```python
from build123d import *

# Parameters (mm, degrees)
SKETCH2_R           = 15
SKETCH2_R_2         = 12.5
BOSS_EXTRUDE1_DEPTH = 35
SKETCH3_R           = 15
BOSS_EXTRUDE2_DEPTH = 5
SKETCH4_W           = 22.056214186
SKETCH4_H           = 2.649940184
BOSS_EXTRUDE3_DEPTH = 10
SKETCH5_W           = 4.385639536
SKETCH5_H           = 22.056214186
BOSS_EXTRUDE4_DEPTH = 40
FILLET1_R           = 2.5


with BuildPart() as part:
    # Sketch2 → Boss-Extrude1 (new body)
    with BuildSketch(Plane(origin=(0, 0, 0), x_dir=(1, 0, 0), z_dir=(0, 1, 0))):
        with Locations(Location((0, 0, 0), (0, 0, 270))):
            Circle(SKETCH2_R)
        with Locations(Location((0, 0, 0), (0, 0, 270))):
            Circle(SKETCH2_R_2, mode=Mode.SUBTRACT)
    extrude(amount=BOSS_EXTRUDE1_DEPTH)

    # Sketch3 → Boss-Extrude2 (add)
    with BuildSketch(Plane(origin=(0, 35, 0), x_dir=(1, 0, 0), z_dir=(0, 1, 0))):
        with Locations(Location((0, 0, 0), (0, 0, 270))):
            Circle(SKETCH3_R)
    extrude(amount=BOSS_EXTRUDE2_DEPTH)

    # Sketch4 → Boss-Extrude3 (add)
    with BuildSketch(Plane(origin=(10, 0, 0), x_dir=(0, 0, -1), z_dir=(1, 0, 0))):
        with Locations((0, 37.460010141)):
            Rectangle(SKETCH4_W, SKETCH4_H)
    extrude(amount=BOSS_EXTRUDE3_DEPTH)

    # Sketch5 → Boss-Extrude4 (add)
    with BuildSketch(Plane.XZ.offset(-36.135040049)):
        with Locations((17.807180232, 0)):
            Rectangle(SKETCH5_W, SKETCH5_H)
    extrude(amount=BOSS_EXTRUDE4_DEPTH)

    # Fillet1
    fillet1_edges = [part.edges().sort_by_distance(p)[0] for p in [
        (20, 17.460010141, -11.028107093),
        (20, 38.784980233, 0),
        (20, 17.460010141, 11.028107093),
        (20, -3.864959951, 0),
    ]]
    fillet(fillet1_edges, radius=FILLET1_R)


solid = part.part
```
Build history of the part. All positions in model axes, mm. A direction names the side the tool comes from. Round coordinates to 2 decimals unless told otherwise and drop trailing zeros. Write each loop counter-clockwise with the first axis right and the second up, starting at its lowest first coordinate (ties: lowest second). Pieces come first, ordered by that corner, then holes. Notation, with made-up numbers: (-26.75, 20) - (-17.75, 20) arc R27 cw to (-17.75, 43) - close; hole circle Ø11 at (-2, 87). An arc over 180 degrees is marked (long way). Write each question's results on one line, items separated by ' | '. Start each with the question number.
Item 1: Saw through at D-D (x = 13.5). Write the cut outline in (y, z).
Item 2: Saw through at B-B (x = 0). Write the cut outline in (y, z), and give its area (3 significant figures).
Item 3: Saw through at A-A (y = 5). Write the cut outline in (x, z), and give its area (3 significant figures).
Item 4: Drop flat-ended pins along their axis: P1, Ø1.6, axis at x = 12.5, z = -3.5, coming from the -Y side; P2, Ø1.5, axis at y = 9.5, z = 10, coming from the +X side; P3, Ø1, axis at x = 15.5, z = -1, coming from the +Y side (3 decimals); P4, Ø12, axis at y = 12.5, z = -5, coming from the -X side. Give the stop position or say it passes through.
Item 5: Saw through at C-C (z = 0). Write the cut outline in (x, y), and give its area (3 significant figures).
Item 6: Which spindle directions (+Z, -Z, +X, -X, +Y, -Y) get a long thin tool onto all of the face, cutting with end or side? Do faces 1 (the face through (15.614, 16, 0)), 2 (the face through (17, 21, 11.028)), 3 (the face through (3.755, 17.255, 11.923)). Say none if no direction does.
Item 7: Wall check: L1, parallel to X at y = 21, z = 0; L2, parallel to X at y = 17, z = -6.75; L3, parallel to Z at x = -0.5, y = 13.5. Give the ranges that are in metal, low to high. Write a range as [from, to].
Results are:
1) outline: (0, -6.54) - (36.14, -6.54) - (36.14, -11.03) - (38.78, -11.03) - (38.78, -6.54) - (40, -6.54) - (40, 6.54) - (38.78, 6.54) - (38.78, 11.03) - (36.14, 11.03) - (36.14, 6.54) - (0, 6.54) - close
2) outline: (0, -15) - (40, -15) - (40, 15) - (0, 15) - (0, 12.5) - (35, 12.5) - (35, -12.5) - (0, -12.5) - close | area: 325 mm²
3) outline: circle Ø30 at (0, 0); (15.61, -11.03) - (17.5, -11.03) arc R2.5 ccw to (20, -8.53) - (20, 8.53) arc R2.5 ccw to (17.5, 11.03) - (15.61, 11.03) - close; hole circle Ø25 at (0, 0) | area: 310 mm²
4) P1: stops at y = 0 | P2: stops at x = 19.89 | P3: stops at y = 38.785 | P4: stops at x = -15
5) outline: (-15, 0) - (-12.5, 0) - (-12.5, 35) - (12.5, 35) - (12.5, 0) - (15, 0) - (15, 36.14) - (15.61, 36.14) - (15.61, -3.86) - (17.5, -3.86) arc R2.5 ccw to (20, -1.36) - (20, 36.28) arc R2.5 ccw to (17.5, 38.78) - (15, 38.78) - (15, 40) - (-15, 40) - close | area: 511 mm²
6) face 1: +Z, -Z, -Y | face 2: +Z, +X, +Y, -Y | face 3: -Y
7) L1: x = [-15, -12.5], [12.5, 15], [15.61, 20] | L2: x = [-13.4, -10.52], [10.52, 13.4], [15.61, 20] | L3: z = [-14.99, -12.49], [12.49, 14.99]
